```python
from build123d import *

# Parameters (mm, degrees)
SKETCH1_W           = 26
SKETCH1_H           = 31
SKETCH1_R           = 5
SKETCH1_R_2         = 2
BOSS_EXTRUDE1_DEPTH = 1.5
SKETCH2_W           = 26
SKETCH2_H           = 1.5
BOSS_EXTRUDE2_DEPTH = 31.5
SKETCH3_R           = 1.6
SKETCH3_R_2         = 4
CUT_EXTRUDE1_DEPTH  = 1.5
FILLET1_R           = 1
FILLET2_R           = 3


with BuildPart() as part:
    # Sketch1 → Boss-Extrude1 (new body)
    with BuildSketch(Plane(origin=(0, 0, 0), x_dir=(1, 0, 0), z_dir=(0, 1, 0))):
        Rectangle(SKETCH1_W, SKETCH1_H)
        with Locations(Location((0, 0, 0), (0, 0, 270))):
            Circle(SKETCH1_R, mode=Mode.SUBTRACT)
        with Locations(Location((-8, 7, 0), (0, 0, 270))):
            Circle(SKETCH1_R_2, mode=Mode.SUBTRACT)
        with Locations(Location((8, 7, 0), (0, 0, 270))):
            Circle(SKETCH1_R_2, mode=Mode.SUBTRACT)
        with Locations(Location((-8, -7, 0), (0, 0, 270))):
            Circle(SKETCH1_R_2, mode=Mode.SUBTRACT)
        with Locations(Location((8, -7, 0), (0, 0, 270))):
            Circle(SKETCH1_R_2, mode=Mode.SUBTRACT)
    extrude(amount=BOSS_EXTRUDE1_DEPTH)

    # Sketch2 → Boss-Extrude2 (add)
    with BuildSketch(Plane(origin=(0, 1.5, 0), x_dir=(1, 0, 0), z_dir=(0, 1, 0))):
        with Locations((0, 14.75)):
            Rectangle(SKETCH2_W, SKETCH2_H)
    extrude(amount=BOSS_EXTRUDE2_DEPTH)

    # Sketch3 → Cut-Extrude1 (cut)
    with BuildSketch(Plane.XY.offset(-14)):
        with BuildLine():
            Line((-13, 33), (-13, 20))
            ThreePointArc((-13, 20), (-9.192388155, 29.192388155), (0, 33))
            Line((0, 33), (-13, 33))
        make_face()
        with BuildLine():
            Line((13, 33), (0, 33))
            ThreePointArc((0, 33), (9.192388155, 29.192388155), (13, 20))
            Line((13, 20), (13, 33))
        make_face()
        with Locations((-8.5, 20)):
            Circle(SKETCH3_R)
        with Locations((0, 20)):
            Circle(SKETCH3_R_2)
        with Locations((8.5, 20)):
            Circle(SKETCH3_R)
    extrude(amount=-CUT_EXTRUDE1_DEPTH, mode=Mode.SUBTRACT)

    # Fillet1
    fillet1_edges = [part.edges().sort_by_distance(p)[0] for p in [
        (0, 1.5, -14),
        (0, 0, -15.5),
    ]]
    fillet(fillet1_edges, radius=FILLET1_R)

    # Fillet2
    fillet2_edges = [part.edges().sort_by_distance(p)[0] for p in [
        (13, 0.75, 15.5),
        (-13, 0.75, 15.5),
    ]]
    fillet(fillet2_edges, radius=FILLET2_R)


solid = part.part
```
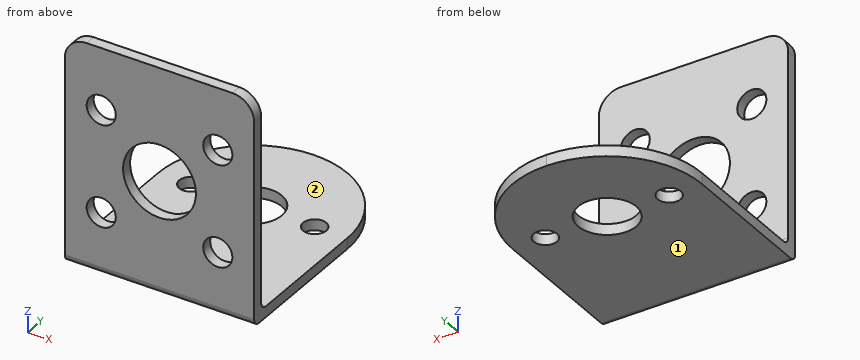
Design review of the part built by this model. Coordinates are the model's own, in mm. Face numbers are marked on the shaded views. A direction names the side the tool comes from. Round coordinates to 2 decimals unless told otherwise and drop trailing zeros. Write each loop counter-clockwise with the first axis right and the second up, starting at its lowest first coordinate (ties: lowest second). Pieces come first, ordered by that corner, then holes. Notation, with made-up numbers: (40, 5.5) -> (82, 5.5) arc R20 ccw to (82, 23.5) -> close; hole circle Ø5 at (52, 6). An arc over 180 degrees is marked (long way). Write item = value, one per line. Start each with the question number.
1) Tool access review of the marked faces 1 and 2: name each direction out of +Z, -Z, +X, -X, +Y, -Y from which nothing blocks a thin tool from reaching the whole face with its end or side.
2) Take a section at D-D, the plane y = 3. State the section outline as (x, z) points, plus the area to 3 significant figures.
3) Wall thickness on probe 1 along X at (y, z) = (1, -7); probe 2 along Y at (x, z) = (-10, 9); probe 3 along Z at (x, y) = (-1, 28): over which ranges is each line inside the solid? List them lowest first. Write a range as from..to.
4) Take a section at C-C, the plane z = 0. State the section outline as (x, y) points, plus the area to 3 significant figures.
5) Take a section at A-A, the plane z = 7. State the section outline as (x, y) points, plus the area to 3 significant figures.
6) Clearance check with flat-ended pins moving along their axes: pin 1 (2.5 mm diameter, centred on x = -8.5, y = 20, fed in from -Z); pin 2 (5 mm diameter, centred on x = -1.5, y = 24, fed in from +Z); pin 3 (4.5 mm diameter, centred on x = -8, z = 7, fed in from +Y); pin 4 (10 mm diameter, centred on y = 11, z = -10, fed in from -X). State where each tip first meets the part, or that it passes through.
7) Take a section at B-B, the plane x = -9.5. State the section outline as (y, z) points.
Results list:
q1.face_1 = -Z, +X, -X, +Y, -Y
q1.face_2 = +Z, +X, -X, +Y
q2.outline = (-13, -15.5) -> (13, -15.5) -> (13, -14) -> (-13, -14) -> close
q2.area = 39.0 mm²
q3.probe_1 = -13..-10, -6..6, 10..13
q3.probe_2 = 0..1.5
q3.probe_3 = -15.5..-14
q4.outline = (-13, 0) -> (-5, 0) -> (-5, 1.5) -> (-13, 1.5) -> close; (5, 0) -> (13, 0) -> (13, 1.5) -> (5, 1.5) -> close
q4.area = 24.0 mm²
q5.outline = (-13, 0) -> (-10, 0) -> (-10, 1.5) -> (-13, 1.5) -> close; (-6, 0) -> (6, 0) -> (6, 1.5) -> (-6, 1.5) -> close; (10, 0) -> (13, 0) -> (13, 1.5) -> (10, 1.5) -> close
q5.area = 27.0 mm²
q6.pin_1 = through
q6.pin_2 = -14
q6.pin_3 = 1.5
q6.pin_4 = -13
q7.outline = (0, -14.5) arc R1 ccw to (1, -15.5) -> (18.75, -15.5) -> (18.75, -14) -> (2.5, -14) arc R1 cw to (1.5, -13) -> (1.5, -8.32) -> (0, -8.32) -> close; (0, -5.68) -> (1.5, -5.68) -> (1.5, 5.68) -> (0, 5.68) -> close; (0, 8.32) -> (1.5, 8.32) -> (1.5, 15.5) -> (0, 15.5) -> close; (21.25, -15.5) -> (28.87, -15.5) -> (28.87, -14) -> (21.25, -14) -> close
